Source: CAD feature listing. Evaluate the final solid. Frame: model axes, mm. A direction names the side the tool comes from. Give positions to 0.01 mm unless a question says otherwise; leave off trailing zeros. Order: outer loops, then holes, each group sorted by start corner. A loop starts at its lowest first (then second) coordinate and runs counter-clockwise, first axis right, second up.
```python
from build123d import *

# Parameters (mm, degrees)
SKETCH2_W           = 38.1
SKETCH2_H           = 6.35
BOSS_EXTRUDE1_DEPTH = 7.62
SKETCH3_W           = 5.08
SKETCH3_H           = 7.62
BOSS_EXTRUDE2_DEPTH = 12.7
SKETCH4_W           = 5.08
SKETCH4_H           = 4.445
BOSS_EXTRUDE3_DEPTH = 11.43
CUT_EXTRUDE2_DEPTH  = 43.828384571
FILLET1_R           = 2.54
SKETCH8_R           = 0.5334
CUT_EXTRUDE4_DEPTH  = 28.305


with BuildPart() as part:
    # Sketch2 → Boss-Extrude1 (new body)
    with BuildSketch(Plane(origin=(0, 0, 0), x_dir=(1, 0, 0), z_dir=(0, 1, 0))):
        Rectangle(SKETCH2_W, SKETCH2_H)
    extrude(amount=BOSS_EXTRUDE1_DEPTH)

    # Sketch3 → Boss-Extrude2 (add)
    with BuildSketch(Plane(origin=(0, 0, -3.175), x_dir=(-1, 0, 0), z_dir=(0, 0, -1))):
        with Locations((-16.51, 3.81)):
            Rectangle(SKETCH3_W, SKETCH3_H)
    boss_extrude2 = extrude(amount=BOSS_EXTRUDE2_DEPTH)

    # Mirror1: Boss-Extrude2 across plane
    add(boss_extrude2.mirror(Plane.XY))

    # Sketch4 → Boss-Extrude3 (add)
    with BuildSketch(Plane.XZ):
        with Locations((16.51, 13.6525)):
            Rectangle(SKETCH4_W, SKETCH4_H)
        with Locations((16.51, -13.6525)):
            Rectangle(SKETCH4_W, SKETCH4_H)
    extrude(amount=BOSS_EXTRUDE3_DEPTH)

    # Sketch6 → Cut-Extrude2 (cut, through all)
    with BuildSketch(Plane(origin=(19.05, 0, 0), x_dir=(0, 0, -1), z_dir=(1, 0, 0))):
        with BuildLine():
            ThreePointArc((-14.991025404, -5.45), (-15.125, -5.95), (-14.991025404, -6.45))
            ThreePointArc((-14.991025404, -6.45), (-13.866180955, -6.915925826), (-13.125, -5.95))
            ThreePointArc((-13.125, -5.95), (-13.866180955, -4.984074174), (-14.991025404, -5.45))
        make_face()
        with BuildLine():
            ThreePointArc((15.125, -5.95), (15.090925826, -5.691180955), (14.991025404, -5.45))
            ThreePointArc((14.991025404, -5.45), (13.125, -5.95), (14.991025404, -6.45))
            ThreePointArc((14.991025404, -6.45), (15.090925826, -6.208819045), (15.125, -5.95))
        make_face()
    extrude(amount=-CUT_EXTRUDE2_DEPTH, mode=Mode.SUBTRACT)

    # Fillet1
    fillet1_edges = [part.edges().sort_by_distance(p)[0] for p in [
        (13.97, 3.81, -3.175),
        (16.51, 7.62, -15.875),
        (16.51, 7.62, 15.875),
        (13.97, 3.81, 3.175),
        (16.51, -11.43, 15.875),
        (16.51, -11.43, -15.875),
        (-19.05, 3.81, 3.175),
        (-19.05, 3.81, -3.175),
    ]]
    fillet(fillet1_edges, radius=FILLET1_R)

    # Sketch8 → Cut-Extrude4 (cut, through all)
    with BuildSketch(Plane.XZ):
        with Locations(Location((-0.85725, 0, 0), (0, 0, 270))):
            Circle(SKETCH8_R)
        with Locations(Location((-9.36625, 0, 0), (0, 0, 270))):
            Circle(SKETCH8_R)
    extrude(amount=-CUT_EXTRUDE4_DEPTH, mode=Mode.SUBTRACT)


solid = part.part
```
1) Material intervals for L1, parallel to X at y = 3.75, z = 0; L2, parallel to Z at x = 17.65, y = -5.95 (3 decimals); L3, parallel to Y at x = 14.5, z = -4, sorted ascending.
Report:
L1: x = -19.05 to -9.9, -8.83 to -1.39, -0.32 to 19.05
L2: z = -15.875 to -15.125, -13.125 to -11.43, 11.43 to 13.125, 15.125 to 15.875
L3: y = 0 to 7.62
2) Section query C-C, the plane x = -5. Return the cut outline in (y, z) (3 decimals).
Report:
outline: (0, -3.175) - (7.62, -3.175) - (7.62, 3.175) - (0, 3.175) - close
3) Section query D-D, the plane z = 8.5. Return the cut outline in (x, y).
Report:
outline: (13.97, 0) - (19.05, 0) - (19.05, 7.62) - (13.97, 7.62) - close
4) Pin query (flat end, axial travel): pin 1 (8 mm diameter, centred on x = 5.5, z = 9.5, fed in from +Y); pin 2 (6 mm diameter, centred on x = -5.5, y = 3, fed in from +Z) (3 decimals); pin 3 (8 mm diameter, centred on y = -5, z = -13.5, fed in from -X); pin 4 (11.5 mm diameter, centred on x = -4.5, z = -3.5, fed in from -Y). Return the tip coordinate at first contact, or that it passes through.
Report:
pin 1: passes through
pin 2: stops at z = 3.175
pin 3: stops at x = 13.97
pin 4: stops at y = 0
5) Reachability of faces 1 (the flat face through (16, -6, 11.43)), 2 (the flat face through (5, 7.62, 0)), 3 (the flat face through (13.97, 0, 12)), 4 (the flat face through (-3, 4, -3.175)), 5 (the flat face through (16, -11.43, 12)) from +Z, -Z, +X, -X, +Y, -Y: full face, straight path, thin tool, end or side. Return the list, or none.
Report:
face 1: +X, -X, -Y
face 2: +Z, -Z, +X, -X, +Y
face 3: +Z, -X, +Y, -Y
face 4: -Z, -X, +Y, -Y
face 5: +Z, -Z, +X, -X, -Y
6) Draft query along Z for faces 6 (the cylindrical face through (-18.286, 3.863, 2.451)), 7 (the flat face through (16, -6, -11.43)), 8 (the flat face through (-19.05, 4, 0)), 9 (the cylindrical face through (16, 7, -15)). Return one class per face: +Z half, -Z half, draft (parallel to the pull), parting line (faces both ways), or undercut.
Report:
face 6: +Z half
face 7: undercut
face 8: draft
face 9: -Z half
7) Section query A-A, the plane y = -2.5. Return the cut outline in (x, z) (3 decimals), and give its area (3 significant figures).
Report:
outline: (13.97, -15.875) - (19.05, -15.875) - (19.05, -11.43) - (13.97, -11.43) - close; (13.97, 11.43) - (19.05, 11.43) - (19.05, 15.875) - (13.97, 15.875) - close
area: 45.2 mm2
8) Section query B-B, the plane z = 0. Return the cut outline in (x, y), and give its area (3 significant figures).
Report:
outline: (-19.05, 0) - (-9.9, 0) - (-9.9, 7.62) - (-19.05, 7.62) - close; (-8.83, 0) - (-1.39, 0) - (-1.39, 7.62) - (-8.83, 7.62) - close; (-0.32, 0) - (19.05, 0) - (19.05, 7.62) - (-0.32, 7.62) - close
area: 274 mm2
